Build history of the part. All positions in model axes, mm. Face numbers are marked on the shaded views. A direction names the side the tool comes from. Coordinates: 2 decimals unless noted, no trailing zeros. Loops run counter-clockwise (first coordinate to the right, second up) from the corner with the lowest first, then second, coordinate; pieces in that order, holes last.
(1) Slice it at A-A (y = 12.25). Give the cut face in (x, z) (3 decimals), and give its area (3 significant figures).
(2) Two-plate mould, pull along Y, no slides. Class the marked faces 4, 5 and 6: pulls with the +Y half, pulls with the -Y half, needs draft (parallel to the pull), parting line crosses it, or undercut.
(3) Slice it at D-D (y = 9.5). Give the cut face in (x, z) (3 decimals).
(4) Wall check: L1, parallel to Z at x = 0, y = 7.25; L2, parallel to Z at x = 1, y = 18.5; L3, parallel to Y at x = -0.5, z = 4. Give the ranges that are in metal, low to high.
(5) Slice it at C-C (z = 1.25). Give the cut face in (x, y) (3 decimals), and give its area (3 significant figures).
(6) Slice it at B-B (x = 22). Give the cut face in (y, z), and give its area (3 significant figures).
(7) Flat gauge pin, fed straight in: P1, Ø1.6, axis at y = 16.5, z = -1.5, coming from the -X side (3 decimals). Where does the tip first touch, or does it go through?
(8) Tool access for the marked faces 1, 2 and 3: list every direction of +Z, -Z, +X, -X, +Y, -Y with a clear straight run to the whole face (end or side of a thin tool).
from build123d import *

# Parameters (mm, degrees)
SKETCH2_W           = 54.25
SKETCH2_H           = 24.5
BOSS_EXTRUDE1_DEPTH = 2
BOSS_EXTRUDE2_DEPTH = 15.5
SKETCH5_W           = 54.25
SKETCH5_H           = 24.5
BOSS_EXTRUDE3_DEPTH = 2
SKETCH6_W           = 11.5
SKETCH6_H           = 6.5
SKETCH6_H_2         = 2
BOSS_EXTRUDE4_DEPTH = 51.5
SKETCH8_W           = 50.25
SKETCH8_H           = 4.3
CUT_EXTRUDE1_DEPTH  = 37.350077373
SKETCH9_W           = 11.5
SKETCH9_H           = 2
CUT_EXTRUDE2_DEPTH  = 5
SKETCH10_W          = 8
SKETCH10_H          = 5
CUT_EXTRUDE3_DEPTH  = 5
FILLET1_R           = 0.5
FILLET2_R           = 1


with BuildPart() as part:
    # Sketch2 → Boss-Extrude1 (new body)
    with BuildSketch(Plane(origin=(0, 0, 0), x_dir=(1, 0, 0), z_dir=(0, 1, 0))):
        with Locations((1, 0)):
            Rectangle(SKETCH2_W, SKETCH2_H)
    extrude(amount=BOSS_EXTRUDE1_DEPTH)

    # Sketch3 → Boss-Extrude2 (add)
    with BuildSketch(Plane(origin=(0, 2, 0), x_dir=(1, 0, 0), z_dir=(0, 1, 0))):
        Polygon((-26.125, 12.25), (28.125, 12.25), (28.125, -12.25), (-26.125, -12.25), (-26.125, -9.5), (25.375, -9.5), (25.375, 9.5), (-26.125, 9.5), align=None)
    extrude(amount=BOSS_EXTRUDE2_DEPTH)

    # Sketch5 → Boss-Extrude3 (add)
    with BuildSketch(Plane(origin=(0, 17.5, 0), x_dir=(1, 0, 0), z_dir=(0, 1, 0))):
        with Locations((1, 0)):
            Rectangle(SKETCH5_W, SKETCH5_H)
    extrude(amount=BOSS_EXTRUDE3_DEPTH)

    # Sketch6 → Boss-Extrude4 (add)
    with BuildSketch(Plane.ZY.offset(-25.375)):
        with Locations((0, 5.25)):
            Rectangle(SKETCH6_W, SKETCH6_H)
        with Locations((0, 16.5)):
            Rectangle(SKETCH6_W, SKETCH6_H_2)
    extrude(amount=BOSS_EXTRUDE4_DEPTH)

    # Sketch8 → Cut-Extrude1 (cut, through all)
    with BuildSketch(Plane(origin=(0, 19.5, 0), x_dir=(1, 0, 0), z_dir=(0, 1, 0))):
        with Locations((0, 7.1)):
            Rectangle(SKETCH8_W, SKETCH8_H)
        with Locations((0, -7.1)):
            Rectangle(SKETCH8_W, SKETCH8_H)
    extrude(amount=-CUT_EXTRUDE1_DEPTH, mode=Mode.SUBTRACT)

    # Sketch9 → Cut-Extrude2 (cut)
    with BuildSketch(Plane.ZY.offset(26.125)):
        with Locations((0, 16.5)):
            Rectangle(SKETCH9_W, SKETCH9_H)
    extrude(amount=-CUT_EXTRUDE2_DEPTH, mode=Mode.SUBTRACT)

    # Sketch10 → Cut-Extrude3 (cut)
    with BuildSketch(Plane.ZY.offset(-25.375)):
        with Locations((0, 13)):
            Rectangle(SKETCH10_W, SKETCH10_H)
    extrude(amount=-CUT_EXTRUDE3_DEPTH, mode=Mode.SUBTRACT)

    # Fillet1
    fillet1_edges = [part.edges().sort_by_distance(p)[0] for p in [
        (-25.125, 18.5, -9.25),
        (25.125, 18.5, -9.25),
        (25.125, 4.25, -4.95),
        (25.125, 17.5, -4.95),
        (-25.125, 4.25, -4.95),
        (-25.125, 1, -9.25),
        (25.125, 1, -9.25),
        (25.125, 18.5, 9.25),
        (-25.125, 4.25, 4.95),
        (25.125, 17.5, 4.95),
        (-25.125, 18.5, 9.25),
        (25.125, 4.25, 4.95),
        (25.125, 1, 9.25),
        (-25.125, 1, 9.25),
        (-25.125, 18.5, -4.95),
        (-25.125, 18.5, 4.95),
        (26.75, 10.5, -4),
        (26.75, 15.5, -4),
        (26.75, 15.5, 4),
        (26.75, 10.5, 4),
    ]]
    fillet(fillet1_edges, radius=FILLET1_R)

    # Fillet2
    fillet2_edges = [part.edges().sort_by_distance(p)[0] for p in [
        (-26.125, 19.5, 0),
        (1, 19.5, 12.25),
        (28.125, 19.5, 0),
        (1, 19.5, -12.25),
        (28.125, 0, 0),
        (1, 0, 12.25),
        (-26.125, 0, 0),
        (1, 0, -12.25),
        (28.125, 9.75, -12.25),
        (28.125, 9.75, 12.25),
        (-26.125, 9.75, 12.25),
        (-26.125, 9.75, -12.25),
    ]]
    fillet(fillet2_edges, radius=FILLET2_R - 0.0001)  # a hair under: the kernel refuses the full size


solid = part.part
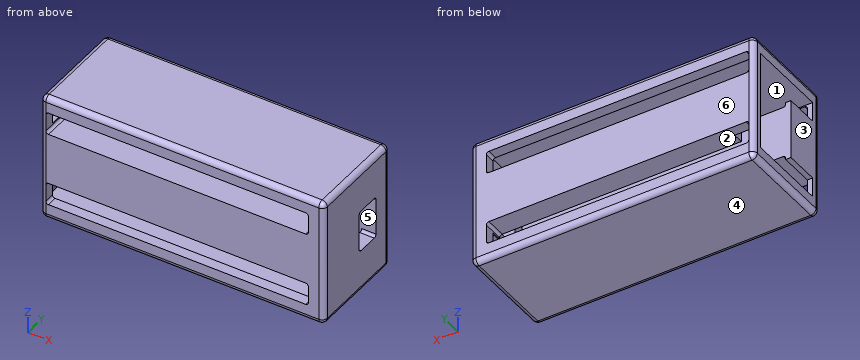
Response values:
1. outline: (-26.125, -11.25) arc R1 ccw to (-25.125, -12.25) - (27.125, -12.25) arc R1 ccw to (28.125, -11.25) - (28.125, -4) - (25.375, -4) - (25.375, -9.5) - (-26.125, -9.5) - close; (-26.125, 9.5) - (25.375, 9.5) - (25.375, 4) - (28.125, 4) - (28.125, 11.25) arc R1 ccw to (27.125, 12.25) - (-25.125, 12.25) arc R1 ccw to (-26.125, 11.25) - close
1. area: 328 mm2
2. face 4: needs draft
2. face 5: undercut
2. face 6: pulls with the +Y half
3. outline: (-26.125, -11.25) arc R1 ccw to (-25.125, -12.25) - (27.125, -12.25) arc R1 ccw to (28.125, -11.25) - (28.125, 11.25) arc R1 ccw to (27.125, 12.25) - (-25.125, 12.25) arc R1 ccw to (-26.125, 11.25) - (-26.125, 9.5) - (25.375, 9.5) - (25.375, -9.5) - (-26.125, -9.5) - close
4. L1: z = -12.25 to -9.5, -4.95 to 4.95, 9.5 to 12.25
4. L2: z = -12.25 to -9.25, -4.95 to 4.95, 9.25 to 12.25
4. L3: y = 0 to 8.5, 15.5 to 19.5
5. outline: (-26.125, 1) arc R1 ccw to (-25.125, 0) - (27.125, 0) arc R1 ccw to (28.125, 1) - (28.125, 10.5) - (25.375, 10.5) - (25.375, 8.5) - (-26.125, 8.5) - close; (-26.125, 17.5) - (-21.125, 17.5) - (-21.125, 15.5) - (28.125, 15.5) - (28.125, 18.5) arc R1 ccw to (27.125, 19.5) - (-25.125, 19.5) arc R1 ccw to (-26.125, 18.5) - close
5. area: 673 mm2
6. outline: (0, -11.25) arc R1 ccw to (1, -12.25) - (18.5, -12.25) arc R1 ccw to (19.5, -11.25) - (19.5, -9.25) - (17.5, -9.25) - (17.5, -9.5) - (2, -9.5) - (2, -9.25) - (0, -9.25) - close; (0, -4.95) - (8.5, -4.95) - (8.5, 4.95) - (0, 4.95) - close; (0, 9.25) - (2, 9.25) - (2, 9.5) - (17.5, 9.5) - (17.5, 9.25) - (19.5, 9.25) - (19.5, 11.25) arc R1 ccw to (18.5, 12.25) - (1, 12.25) arc R1 ccw to (0, 11.25) - close; (15.5, -4.95) - (19.5, -4.95) - (19.5, 4.95) - (15.5, 4.95) - close
6. area: 232 mm2
7. P1: stops at x = -21.125
8. face 1: -X
8. face 2: +Y, -Y
8. face 3: +Z, -Z, -X, +Y, -Y
